Part model, mm, in its own coordinate system. Face numbers are marked on the shaded views. Coordinates: 2 decimals unless noted, no trailing zeros. Loops run counter-clockwise (first coordinate to the right, second up) from the corner with the lowest first, then second, coordinate; pieces in that order, holes last. Notation, with made-up numbers: (81, 34.25) - (116, 34.25) arc R24 cw to (116, 49.25) - close; hole circle Ø7 at (48.25, 70). An arc over 180 degrees is marked (long way). Use a Markdown table: item, result. Add a question column.
1. Band-saw the part on A-A, the plane z = -2. Give the cut face in (x, y), plus the area to 3 significant figures.
2. Pull direction X, two halves, no side cores. Call the marked faces 1 and 2: pulls with the +X half, pulls with the -X half, needs draft (parallel to the pull), parting line crosses it, or undercut.
3. Drop flat-ended pins along their axis: pin 1 (2 mm diameter, centred on x = 1.5, z = 8.5, fed in from +Y); pin 2 (1.5 mm diameter, centred on y = -1.5, z = 6, fed in from +X). Give the stop position or say it passes through.
4. Wall check: probe 1 along Z at (x, y) = (-1.15, 0.8); probe 2 along Z at (x, y) = (2.15, 0.05); probe 3 along Y at (x, z) = (0.2, 1.75). Give the ranges that are in metal, low to high. Write a range as [from, to].
5. Band-saw the part on D-D, the plane z = 2.25. Give the cut face in (x, y).
6. Band-saw the part on B-B, the plane y = 0. Give the cut face in (x, z).
7. Band-saw the part on C-C, the plane z = 6.75. Give the cut face in (x, y), plus the area to 3 significant figures.
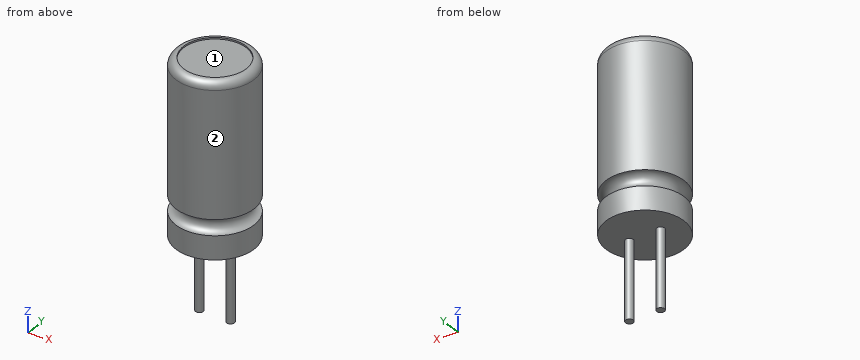
from build123d import *

# Parameters (mm, degrees)
SKETCH3_R           = 2
CUT_EXTRUDE1_DEPTH  = 0.1
SKETCH4_R           = 0.25
BOSS_EXTRUDE1_DEPTH = 5


with BuildPart() as part:
    # Sketch2 → Base-Revolve (revolve)
    with BuildSketch(Plane(origin=(0, 0, 0), x_dir=(0, 0, -1), z_dir=(1, 0, 0))):
        with BuildLine():
            Line((0, 0), (0, 2.5))
            Line((0, 2.5), (-1.5, 2.5))
            ThreePointArc((-1.5, 2.5), (-2, 2), (-2.5, 2.5))
            Line((-2.5, 2.5), (-10.5, 2.5))
            ThreePointArc((-10.5, 2.5), (-10.853553391, 2.353553391), (-11, 2))
            Line((-11, 2), (-11, 0))
            Line((-11, 0), (0, 0))
        make_face()
    revolve(axis=Axis((0, 0, 11), (0, 0, -1)))

    # Sketch3 → Cut-Extrude1 (cut)
    with BuildSketch(Plane.XY.offset(11)):
        Circle(SKETCH3_R)
    extrude(amount=-CUT_EXTRUDE1_DEPTH, mode=Mode.SUBTRACT)

    # Sketch4 → Boss-Extrude1 (add)
    with BuildSketch(Plane(origin=(0, 0, 0), x_dir=(-1, 0, 0), z_dir=(0, 0, -1))):
        with Locations((1, 0)):
            Circle(SKETCH4_R)
        with Locations((-1, 0)):
            Circle(SKETCH4_R)
    extrude(amount=BOSS_EXTRUDE1_DEPTH)


solid = part.part
Geometry check:
| question | item | result |
|---|---|---|
| 1 | outline | circle Ø0.5 at (-1, 0); circle Ø0.5 at (1, 0) |
| 1 | area | 0.393 mm^2 |
| 2 | face 1 | undercut |
| 2 | face 2 | parting line crosses it |
| 3 | pin 1 | stops at y = 2.45 |
| 3 | pin 2 | stops at x = 2.38 |
| 4 | probe 1 | z = [0, 10.9] |
| 4 | probe 2 | z = [0, 1.64], [2.36, 10.98] |
| 4 | probe 3 | y = [-2.06, 2.06] |
| 5 | outline | circle Ø4.13 at (0, 0) |
| 6 | outline | (-2.5, 0) - (-1.25, 0) - (-1.25, -5) - (-0.75, -5) - (-0.75, 0) - (0.75, 0) - (0.75, -5) - (1.25, -5) - (1.25, 0) - (2.5, 0) - (2.5, 1.5) arc R0.5 cw to (2.5, 2.5) - (2.5, 10.5) arc R0.5 ccw to (2, 11) - (2, 10.9) - (-2, 10.9) - (-2, 11) arc R0.5 ccw to (-2.5, 10.5) - (-2.5, 2.5) arc R0.5 cw to (-2.5, 1.5) - close |
| 7 | outline | circle Ø5 at (0, 0) |
| 7 | area | 19.6 mm^2 |
